from build123d import *

# Parameters (mm, degrees)
CUT_EXTRUDE_1_DEPTH      = 33.787192622
CUT_EXTRUDE_1_DEPTH_BACK = 33.787192622
SKETCH_5_R               = 9
CUT_EXTRUDE_2_DEPTH      = 15
CUT_EXTRUDE_3_DEPTH      = 14


with BuildPart() as part:
    # 草图1 → 旋转2 (revolve)
    with BuildSketch(Plane.XY):
        with BuildLine():
            Line((-10, 25), (-10, 11.180339887))
            ThreePointArc((-10, 11.180339887), (-14.012585384, -5.352331347), (0, -15))
            Line((0, -15), (0, 25))
            Line((0, 25), (-10, 25))
        make_face()
    revolve(axis=Axis((0, 25, 0), (0, -1, 0)))

    # 草图4 → 切除-拉伸1 (cut, two sides: drawn at the far end of the back side and taken through both)
    with BuildSketch(Plane.XY.offset(-CUT_EXTRUDE_1_DEPTH_BACK)):
        with BuildLine():
            ThreePointArc((10.606601718, -10.606601718), (-10.606601718, -10.606601718), (-10.606601718, 10.606601718))
            Line((-10.606601718, 10.606601718), (0, 0))
            Line((0, 0), (10.606601718, -10.606601718))
        make_face()
    extrude(amount=CUT_EXTRUDE_1_DEPTH + CUT_EXTRUDE_1_DEPTH_BACK, mode=Mode.SUBTRACT)

    # 草图5 → 切除-拉伸2 (cut)
    with BuildSketch(Plane(origin=(0, 25, 0), x_dir=(1, 0, 0), z_dir=(0, 1, 0))):
        with Locations(Location((0, 0, 0), (0, 0, 180))):
            Circle(SKETCH_5_R)
    extrude(amount=-CUT_EXTRUDE_2_DEPTH, mode=Mode.SUBTRACT)

    # 草图6 → 切除-拉伸3 (cut)
    with BuildSketch(Plane(origin=(0, 0, 0), x_dir=(0, 0, -1), z_dir=(1, 0, 0))):
        Polygon((0, 12), (4, 12), (4, 15), (-4, 15), (-4, 12), align=None)
    extrude(amount=-CUT_EXTRUDE_3_DEPTH, mode=Mode.SUBTRACT)


solid = part.part
Verification items for the finished model (mm, model axes). A direction names the side the tool comes from. Give positions to 0.01 mm unless a question says otherwise; leave off trailing zeros. Order: outer loops, then holes, each group sorted by start corner. A loop starts at its lowest first (then second) coordinate and runs counter-clockwise, first axis right, second up. Notation, with made-up numbers: M 88.25,41 L 118.25,41 A13 cw 118.25,51 Z; hole C 33,-34.5 d6. An arc over 180 degrees is marked long. Use one line per item in the form item = value. Start each with the question number.
Q1. Access from +Z, -Z, +X, -X, +Y, -Y to the whole of each face (thin tool, end or side, straight path). Record for faces 1 (the cylindrical face through (10, 18, 0)), 2 (the flat face through (-9.2, 15, -0.1)), 3 (the flat face through (-9, 25, -2)).
Q2. Section check A-A (z = 0). Enter the section's corners in (x, y), then the cut area to 3 significant figures.
Q3. Mould release check, pull along X, two halves, no side actions. Record for faces 4 (the flat face through (0, 0, 0)), 5 (the flat face through (0, 10, 0)), 6 (the flat face through (-9.2, 12, 0.1)), 7 (the cylindrical face through (9, 18, 0)): +X half, -X half, draft (parallel to the pull), parting line (faces both ways), or undercut.
Q4. Go/stop test with flat-tipped pins: pin 1 Ø4 at (x, y) = (5, 3.5) entering from -Z; pin 2 Ø1.2 at (x, y) = (-8.5, 13.5) entering from +Z; pin 3 Ø2 at (x, z) = (8.5, 8) entering from -Y. Record where each tip stops, or that it passes through.
Q5. Section check B-B (x = 0). Enter the section's corners in (y, z).
Q6. Section check D-D (y = 13). Enter the section's corners in (x, z), then the cut area to 3 significant figures.
Q7. Scan lines: line 1 along Z through (x, y) = (0, 16.75); line 2 along X through (y, z) = (11, -5); line 3 along X through (y, z) = (18, 6). Record each from-to range of solid material in increasing order. Write a range as [from, to].
Q8. Section check C-C (y = 23). Enter the section's corners in (x, z).
Evaluation:
q1.face_1 = +Y
q1.face_2 = -X
q1.face_3 = +Z, -Z, +X, -X, +Y
q2.outline = M -10.61,10.61 L 10.61,-10.61 A15 ccw 10,11.18 L 10,25 L 9,25 L 9,10 L -9,10 L -9,12 L -10,12 L -10,11.18 A15 ccw Z; M -10,15 L -9,15 L -9,25 L -10,25 Z
q2.area = 304 mm2
q3.face_4 = -X half
q3.face_5 = undercut
q3.face_6 = draft
q3.face_7 = undercut
q4.pin_1 = -14.43
q4.pin_2 = 6.13
q4.pin_3 = -9.25
q5.outline = M 0,-15 A15 ccw 11.18,-10 L 25,-10 L 25,-9 L 10,-9 L 10,9 L 25,9 L 25,10 L 11.18,10 A15 ccw 0,15 Z
q6.outline = M -9.17,-4 A10 ccw long -9.17,4 L -8.06,4 A9 cw long -8.06,-4 Z
q6.area = 51.4 mm2
q7.line_1 = [-10, -9], [9, 10]
q7.line_2 = [-8.89, -7.48], [7.48, 8.89]
q7.line_3 = [-8, -6.71], [6.71, 8]
q8.outline = C 0,0 d20; hole C 0,0 d18
